from build123d import *

# Parameters (mm, degrees)
SKETCH_1_R      = 1.6
EXTRUDE_1_DEPTH = 3


with BuildPart() as part:
    # 草图1 → 凸台-拉伸1 (new body)
    with BuildSketch(Plane.XY):
        Polygon((0, 0), (40, 0), (40, -15), (20, -35), (0, -35), align=None)
        with Locations((5, -30)):
            Circle(SKETCH_1_R, mode=Mode.SUBTRACT)
        with Locations(Location((15, -30, 0), (0, 0, 180))):
            Circle(SKETCH_1_R, mode=Mode.SUBTRACT)
        with Locations((15, -20)):
            Circle(SKETCH_1_R, mode=Mode.SUBTRACT)
        with Locations(Location((5, -20, 0), (0, 0, 180))):
            Circle(SKETCH_1_R, mode=Mode.SUBTRACT)
        with Locations((35, -3.75)):
            Circle(SKETCH_1_R, mode=Mode.SUBTRACT)
        with Locations(Location((35, -11.25, 0), (0, 0, 180))):
            Circle(SKETCH_1_R, mode=Mode.SUBTRACT)
        with Locations((25, -11.25)):
            Circle(SKETCH_1_R, mode=Mode.SUBTRACT)
        with Locations(Location((25, -3.75, 0), (0, 0, 180))):
            Circle(SKETCH_1_R, mode=Mode.SUBTRACT)
        Polygon((19, -16.5), (19, -28.928932188), (31.428932188, -16.5), align=None, mode=Mode.SUBTRACT)
        Polygon((6, -3.5), (14, -3.5), (6, -11.5), align=None, mode=Mode.SUBTRACT)
    extrude(amount=EXTRUDE_1_DEPTH)


solid = part.part
Could you check a few things on this model? Use its own coordinates, in mm. A direction names the side the tool comes from. Coordinates: 2 decimals unless noted, no trailing zeros. Order: outer loops, then holes, each group sorted by start corner. A loop starts at its lowest first (then second) coordinate and runs counter-clockwise, first axis right, second up.
Q1. Suppose I cut it at C-C on y = -30. Please give me the cut outline in (x, z).
Q2. Which directions (+Z, -Z, +X, -X, +Y, -Y) give clear straight access to the entire face, cutting with the end or side of a thin tool? Please do faces 1 (the flat face through (19, -23, 1)), 2 (the flat face through (10, -35, 1)).
Q3. Please list where these lines run through material, in increasing order: L1, parallel to Y at x = 15, z = 0.2; L2, parallel to X at y = -4.5, z = 1.25; L3, parallel to X at y = -6.5, z = 0.9.
Q4. Suppose I cut it at D-D on x = 25. Please give me the cut outline in (y, z).
Q5. Suppose I cut it at B-B on z = 1.5. Give the number of separate pieces and of enclosed holes in the cut face, and give its area (3 significant figures).
Q6. Will this pin go through, and if not, where does the flat tip stop? pin 1 (2.5 mm diameter, centred on x = 15, y = -20, fed in from -Z).
Q7. Suppose I cut it at A-A on y = -7.5. Please give me the cut outline in (x, z).
Answer:
1. outline: (0, 0) - (3.4, 0) - (3.4, 3) - (0, 3) - close; (6.6, 0) - (13.4, 0) - (13.4, 3) - (6.6, 3) - close; (16.6, 0) - (25, 0) - (25, 3) - (16.6, 3) - close
2. face 1: +Z, -Z
2. face 2: +Z, -Z, +X, -X, -Y
3. L1: y = -35 to -31.6, -28.4 to -21.6, -18.4 to 0
3. L2: x = 0 to 6, 13 to 23.59, 26.41 to 33.59, 36.41 to 40
3. L3: x = 0 to 6, 11 to 40
4. outline: (-30, 0) - (-22.93, 0) - (-22.93, 3) - (-30, 3) - close; (-16.5, 0) - (-12.85, 0) - (-12.85, 3) - (-16.5, 3) - close; (-9.65, 0) - (-5.35, 0) - (-5.35, 3) - (-9.65, 3) - close; (-2.15, 0) - (0, 0) - (0, 3) - (-2.15, 3) - close
5. separate pieces: 1
5. enclosed holes: 10
5. area: 1,030 mm2
6. pin 1: passes through
7. outline: (0, 0) - (6, 0) - (6, 3) - (0, 3) - close; (10, 0) - (40, 0) - (40, 3) - (10, 3) - close
